Input: part model. Units: mm. Frame: model coordinates. Face numbers are marked on the shaded views. Coordinates: 2 decimals unless noted, no trailing zeros. Order: outer loops, then holes, each group sorted by start corner. A loop starts at its lowest first (then second) coordinate and runs counter-clockwise, first axis right, second up. Notation, with made-up numbers: (-28.75, 53.25) - (-5.75, 53.25) arc R22 cw to (-5.75, 87.25) - close; hole circle Ø3 at (-3.75, -39.5). An arc over 180 degrees is marked (long way). Use a Markdown table: item, result. Add a question column.
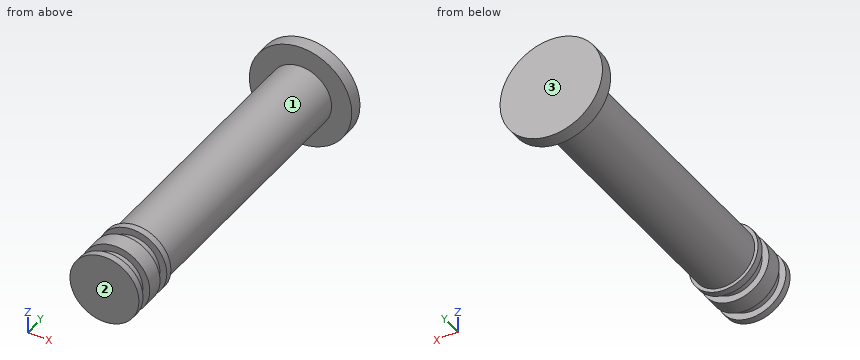
Autodesk Inventor part; units mm, degrees
ref_plane "YZ Plane" through (0, 0, 0) normal (1, 0, 0) x (0, 1, 0)
ref_plane "XZ Plane" through (0, 0, 0) normal (0, 1, 0) x (-1, 0, 0)
ref_plane "XY Plane" through (0, 0, 0) normal (0, 0, 1) x (1, 0, 0)
sketch "Sketch1" plane through (0, 0, 0) normal (0, 1, 0) x (-1, 0, 0)
  circle A0 centre (0, 0) radius 9
  dimension "d0" = 18
extrude "Extrusion1" add sketch "Sketch1" along normal blind 80
sketch "Sketch2" plane through (0, 80, 0) normal (0, 1, 0) x (1, 0, 0)
  circle A0 centre (0, 0) radius 14.85
  dimension "d3" = 29.7
extrude "Extrusion2" add sketch "Sketch2" along normal blind 4
sketch "Sketch3" plane through (0, 0, 0) normal (0, -1, 0) x (1, 0, 0)
  circle A0 centre (0, 0) radius 9
  circle A1 centre (0, 0) radius 10
  dimension "d6" = 20
extrude "Extrusion3" add sketch "Sketch3" along normal blind 2 contours A0 | A1
sketch "Sketch4" plane through (0, -2, 0) normal (0, -1, 0) x (1, 0, 0)
  circle A0 centre (0, 0) radius 8
  dimension "d9" = 16
extrude "Extrusion4" add sketch "Sketch4" along normal blind 3.3
sketch "Sketch5" plane through (0, -5.3, 0) normal (0, -1, 0) x (1, 0, 0)
  circle A0 centre (0, 0) radius 10
  dimension "d12" = 20
extrude "Extrusion5" add sketch "Sketch5" along normal blind 5
sketch "Sketch7" plane through (0, -10.3, 0) normal (0, -1, 0) x (1, 0, 0)
  circle A0 centre (0, 0) radius 8
  dimension "d15" = 16
extrude "Extrusion6" add sketch "Sketch7" along normal blind 3.3
sketch "Sketch8" plane through (0, -13.6, 0) normal (0, -1, 0) x (1, 0, 0)
  circle A0 centre (0, 0) radius 10
  dimension "d18" = 20
extrude "Extrusion7" add sketch "Sketch8" along normal blind 2
properties part number "Plunger"
1) Cut plane C-C (y = 43). Return the cut outline in (x, z).
2) Material intervals for L1, parallel to Y at x = -8.75, z = 3.5; L2, parallel to Y at x = -3.5, z = -7.5; L3, parallel to Y at x = 3, z = 10.5, sorted ascending.
3) Cut plane B-B (z = 0). Return the cut outline in (x, y).
4) Cut plane D-D (y = -1). Return the cut outline in (x, z), and give its area (3 significant figures).
5) Pull-direction query (Y, two-part tool) for the marked faces 1, 2 and 3; classes: pulls with the +Y half, pulls with the -Y half, needs draft (parallel to the pull), parting line crosses it, or undercut.
6) Contact query for flat-ended pins moving along their axis: P1, Ø3, axis at x = -9.5, y = 0.5, coming from the -Z side; P2, Ø8, axis at x = -4.5, y = 64, coming from the +Z side; P3, Ø3, axis at x = -1.5, y = 68, coming from the -Z side. Output: stop coordinate, or through.
7) Cut plane A-A (x = 0). Return the cut outline in (y, z).
Computed:
| question | item | result |
|---|---|---|
| 1 | outline | circle Ø18 at (0, 0) |
| 2 | L1 | y = -15.6 to -13.6, -10.3 to -5.3, -2 to 0, 80 to 84 |
| 2 | L2 | y = -15.6 to -13.6, -10.3 to -5.3, -2 to 84 |
| 2 | L3 | y = 80 to 84 |
| 3 | outline | (-14.85, 80) - (-9, 80) - (-9, 0) - (-10, 0) - (-10, -2) - (-8, -2) - (-8, -5.3) - (-10, -5.3) - (-10, -10.3) - (-8, -10.3) - (-8, -13.6) - (-10, -13.6) - (-10, -15.6) - (10, -15.6) - (10, -13.6) - (8, -13.6) - (8, -10.3) - (10, -10.3) - (10, -5.3) - (8, -5.3) - (8, -2) - (10, -2) - (10, 0) - (9, 0) - (9, 80) - (14.85, 80) - (14.85, 84) - (-14.85, 84) - close |
| 4 | outline | circle Ø20 at (0, 0) |
| 4 | area | 314 mm2 |
| 5 | face 1 | undercut |
| 5 | face 2 | pulls with the -Y half |
| 5 | face 3 | pulls with the +Y half |
| 6 | P1 | stops at z = -5.88 |
| 6 | P2 | stops at z = 8.99 |
| 6 | P3 | stops at z = -9 |
| 7 | outline | (-15.6, -10) - (-13.6, -10) - (-13.6, -8) - (-10.3, -8) - (-10.3, -10) - (-5.3, -10) - (-5.3, -8) - (-2, -8) - (-2, -10) - (0, -10) - (0, -9) - (80, -9) - (80, -14.85) - (84, -14.85) - (84, 14.85) - (80, 14.85) - (80, 9) - (0, 9) - (0, 10) - (-2, 10) - (-2, 8) - (-5.3, 8) - (-5.3, 10) - (-10.3, 10) - (-10.3, 8) - (-13.6, 8) - (-13.6, 10) - (-15.6, 10) - close |
